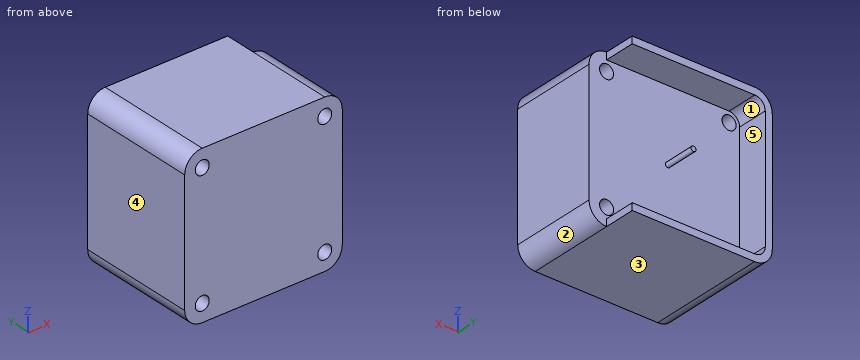
```python
from build123d import *

# Parameters (mm, degrees)
SKETCH1_R           = 4
BOSS_EXTRUDE1_DEPTH = 50
EXTRUDE_THIN1_DEPTH = 18
SKETCH3_R           = 1.4
BOSS_EXTRUDE2_DEPTH = 18
SKETCH4_W           = 4.41201188
SKETCH4_H           = 70
CUT_EXTRUDE1_DEPTH  = 18
SKETCH5_W           = 12.080222771
SKETCH5_H           = 13.922777815
SKETCH5_W_2         = 14.701199749
SKETCH5_H_2         = 17.828925886
CUT_EXTRUDE2_DEPTH  = 18


with BuildPart() as part:
    # Sketch1 → Boss-Extrude1 (new body)
    with BuildSketch(Plane(origin=(0, 0, 0), x_dir=(1, 0, 0), z_dir=(0, 1, 0))):
        with BuildLine():
            Line((-53.889789303, 53.241491086), (16.110210697, 53.241491086))
            ThreePointArc((16.110210697, 53.241491086), (23.181278509, 50.312558898), (26.110210697, 43.241491086))
            Line((26.110210697, 43.241491086), (26.110210697, -26.758508914))
            ThreePointArc((26.110210697, -26.758508914), (23.181278509, -33.829576726), (16.110210697, -36.758508914))
            Line((16.110210697, -36.758508914), (-53.889789303, -36.758508914))
            ThreePointArc((-53.889789303, -36.758508914), (-60.960857115, -33.829576726), (-63.889789303, -26.758508914))
            Line((-63.889789303, -26.758508914), (-63.889789303, 43.241491086))
            ThreePointArc((-63.889789303, 43.241491086), (-60.960857115, 50.312558898), (-53.889789303, 53.241491086))
        make_face()
        with Locations(Location((-53.889789303, 43.241491086, 0), (0, 0, 270))):
            Circle(SKETCH1_R, mode=Mode.SUBTRACT)
        with Locations(Location((16.110210697, 43.241491086, 0), (0, 0, 270))):
            Circle(SKETCH1_R, mode=Mode.SUBTRACT)
        with Locations(Location((16.110210697, -26.758508914, 0), (0, 0, 270))):
            Circle(SKETCH1_R, mode=Mode.SUBTRACT)
        with Locations(Location((-53.889789303, -26.758508914, 0), (0, 0, 270))):
            Circle(SKETCH1_R, mode=Mode.SUBTRACT)
    extrude(amount=BOSS_EXTRUDE1_DEPTH)

    # Sketch2 → Extrude-Thin1 (add)
    with BuildSketch(Plane(origin=(0, 50, 0), x_dir=(1, 0, 0), z_dir=(0, 1, 0))):
        with BuildLine():
            Line((26.110210697, -26.758508914), (26.110210697, 43.241491086))
            ThreePointArc((26.110210697, 43.241491086), (23.181278509, 50.312558898), (16.110210697, 53.241491086))
            Line((16.110210697, 53.241491086), (-53.889789303, 53.241491086))
            ThreePointArc((-53.889789303, 53.241491086), (-60.960857115, 50.312558898), (-63.889789303, 43.241491086))
            Line((-63.889789303, 43.241491086), (-63.889789303, -26.758508914))
            ThreePointArc((-63.889789303, -26.758508914), (-60.960857115, -33.829576726), (-53.889789303, -36.758508914))
            Line((-53.889789303, -36.758508914), (16.110210697, -36.758508914))
            ThreePointArc((16.110210697, -36.758508914), (23.181278509, -33.829576726), (26.110210697, -26.758508914))
        make_face()
        with BuildLine():
            Line((22.110210697, -26.758508914), (22.110210697, 43.241491086))
            ThreePointArc((22.110210697, 43.241491086), (20.352851384, 47.484131773), (16.110210697, 49.241491086))
            Line((16.110210697, 49.241491086), (-53.889789303, 49.241491086))
            ThreePointArc((-53.889789303, 49.241491086), (-58.13242999, 47.484131773), (-59.889789303, 43.241491086))
            Line((-59.889789303, 43.241491086), (-59.889789303, -26.758508914))
            ThreePointArc((-59.889789303, -26.758508914), (-58.13242999, -31.001149601), (-53.889789303, -32.758508914))
            Line((-53.889789303, -32.758508914), (16.110210697, -32.758508914))
            ThreePointArc((16.110210697, -32.758508914), (20.352851384, -31.001149601), (22.110210697, -26.758508914))
        make_face(mode=Mode.SUBTRACT)
    extrude(amount=EXTRUDE_THIN1_DEPTH)

    # Sketch3 → Boss-Extrude2 (add)
    with BuildSketch(Plane(origin=(0, 50, 0), x_dir=(1, 0, 0), z_dir=(0, 1, 0))):
        with Locations(Location((-18.889789303, 8.241491086, 0), (0, 0, 90))):
            Circle(SKETCH3_R)
    extrude(amount=BOSS_EXTRUDE2_DEPTH)

    # Sketch4 → Cut-Extrude1 (cut)
    with BuildSketch(Plane(origin=(0, 68, 0), x_dir=(1, 0, 0), z_dir=(0, 1, 0))):
        with Locations((24.316216637, 8.241491086)):
            Rectangle(SKETCH4_W, SKETCH4_H)
    extrude(amount=-CUT_EXTRUDE1_DEPTH, mode=Mode.SUBTRACT)

    # Sketch5 → Cut-Extrude2 (cut)
    with BuildSketch(Plane(origin=(0, 68, 0), x_dir=(1, 0, 0), z_dir=(0, 1, 0))):
        with Locations((22.150322083, 46.280102179)):
            Rectangle(SKETCH5_W, SKETCH5_H)
        with Locations((23.460810572, -27.844045971)):
            Rectangle(SKETCH5_W_2, SKETCH5_H_2)
    extrude(amount=-CUT_EXTRUDE2_DEPTH, mode=Mode.SUBTRACT)


solid = part.part
```
Here's how the part is built. I have some questions about the finished solid (model axes, mm). Face numbers are marked on the shaded views. A direction names the side the tool comes from. Give positions to 0.01 mm unless a question says otherwise; leave off trailing zeros. Loops run counter-clockwise (first coordinate to the right, second up) from the corner with the lowest first, then second, coordinate; pieces in that order, holes last. Notation, with made-up numbers: M 11.5,-38.5 L 55.5,-38.5 A27 ccw 55.5,-5.5 Z; hole C 76,7.5 d7. An arc over 180 degrees is marked long. Put each result on its own line as item: value. Start each with the question number.
(1) I want a section at A-A on y = 14. Please give me the cut outline in (x, z).
(2) I want a section at B-B on z = -19. Please give me the cut outline in (x, y).
(3) I want a section at D-D on z = -41.5. Please give me the cut outline in (x, y), then the cut area to 3 significant figures.
(4) Will these pins go through, and if not, where does the flat tip stop? pin 1 Ø3 at (y, z) = (62, 34.5) entering from +X; pin 2 Ø20 at (y, z) = (63, -15) entering from +X; pin 3 Ø10.5 at (x, z) = (16.11, -43.24) entering from +Y.
(5) I want a section at C-C on x = -11.5. Please give me the cut outline in (y, z), then the cut area to 3 significant figures.
(6) I need wall thicknesses on line 1 along Z through (x, y) = (-53, 30.5); line 2 along X through (y, z) = (53.5, -6); line 3 along Y through (x, z) = (-35.5, -47). Which ranges of each line are inside material? Lowest first, please. Write a range as [from, to].
(7) For the marked faces 1 and 2, which set-ups out of +Z, -Z, +X, -X, +Y, -Y let a thin tool reach every point of the face, with its end or its side?
(8) If we mould it in two halves opening along Z, with no side actions, what happens to the marked faces 3, 4 and 5? For each: +Z half, -Z half, draft (parallel to the pull), parting line (faces both ways), or undercut.
Answer block:
1. outline: M -63.89,-43.24 A10 ccw -53.89,-53.24 L 16.11,-53.24 A10 ccw 26.11,-43.24 L 26.11,26.76 A10 ccw 16.11,36.76 L -53.89,36.76 A10 ccw -63.89,26.76 Z; hole C -53.89,-43.24 d8; hole C -53.89,26.76 d8; hole C 16.11,-43.24 d8; hole C 16.11,26.76 d8
2. outline: M -63.89,0 L 26.11,0 L 26.11,50 L -59.89,50 L -59.89,68 L -63.89,68 Z
3. outline: M -63.89,0 L -57.49,0 L -57.49,50 L -59.89,50 L -59.89,68 L -63.89,68 Z; M -50.29,0 L 12.51,0 L 12.51,50 L -50.29,50 Z; M 19.71,0 L 26.11,0 L 26.11,50 L 19.71,50 Z
3. area: 3,850 mm^2
4. pin 1: x = 16.11
4. pin 2: x = -17.49
4. pin 3: y = 50
5. outline: M 0,-53.24 L 68,-53.24 L 68,-49.24 L 50,-49.24 L 50,32.76 L 68,32.76 L 68,36.76 L 0,36.76 Z
5. area: 4,640 mm^2
6. line 1: [-53.24, -47.14], [-39.34, 22.86], [30.66, 36.76]
6. line 2: [-63.89, -59.89]
6. line 3: [0, 50]
7. face 1: +X, +Y
7. face 2: -Z, +X, +Y, -Y
8. face 3: -Z half
8. face 4: draft
8. face 5: undercut
